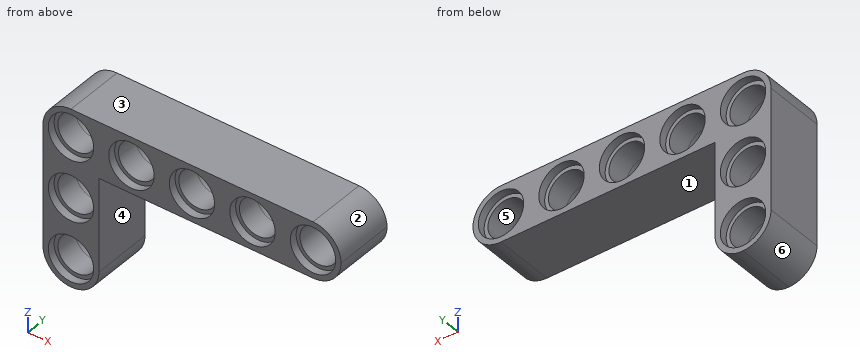
from build123d import *

# Parameters (mm, degrees)
F0_R     = 3
F1_DEPTH = 3.95
F0_R_2   = 2.499
F2_DEPTH = 2.95
F3_R     = 3.69999
F4_R     = 3
F4_W     = 7.4
F4_H     = 7.4
F5_DEPTH = 7.9
F7_R     = 3.69999
F8_R     = 3.7


# Not quite as in the source:
# - a fillet or chamfer is up to 0.001 mm smaller than in the source, because OpenCascade refuses the exact size


with BuildPart() as f1:
    # F0 (on Front) → F1 (new body, symmetric)
    with BuildSketch(Plane.XZ):
        Polygon((19.7, -3.7), (19.7, 3.7), (-19.7, 3.7), (-19.7, -3.7), (-19.7, -19.7), (-12.3, -19.7), (-12.3, -3.7), align=None)
        with Locations((-16, -16)):
            Circle(F0_R, mode=Mode.SUBTRACT)
        with Locations((-16, -8)):
            Circle(F0_R, mode=Mode.SUBTRACT)
        with Locations((-16, 0)):
            Circle(F0_R, mode=Mode.SUBTRACT)
        with Locations((-8, 0)):
            Circle(F0_R, mode=Mode.SUBTRACT)
        Circle(F0_R, mode=Mode.SUBTRACT)
        with Locations((8, 0)):
            Circle(F0_R, mode=Mode.SUBTRACT)
        with Locations((16, 0)):
            Circle(F0_R, mode=Mode.SUBTRACT)
    extrude(amount=F1_DEPTH, both=True)

    # F0 (on Front) → F2 (join, symmetric)
    with BuildSketch(Plane.XZ):
        with Locations((-16, -16)):
            Circle(F0_R)
        with Locations((-16, -16)):
            Circle(F0_R_2, mode=Mode.SUBTRACT)
        with Locations((-16, -8)):
            Circle(F0_R)
        with Locations((-16, -8)):
            Circle(F0_R_2, mode=Mode.SUBTRACT)
        with Locations((-16, 0)):
            Circle(F0_R)
        with Locations((-16, 0)):
            Circle(F0_R_2, mode=Mode.SUBTRACT)
        with Locations((-8, 0)):
            Circle(F0_R)
        with Locations((-8, 0)):
            Circle(F0_R_2, mode=Mode.SUBTRACT)
        Circle(F0_R)
        Circle(F0_R_2, mode=Mode.SUBTRACT)
        with Locations((8, 0)):
            Circle(F0_R)
        with Locations((8, 0)):
            Circle(F0_R_2, mode=Mode.SUBTRACT)
        with Locations((16, 0)):
            Circle(F0_R)
        with Locations((16, 0)):
            Circle(F0_R_2, mode=Mode.SUBTRACT)
    extrude(amount=F2_DEPTH, both=True)

    # F3 (radius 3.7 in the source; OpenCascade refuses exactly that, so slightly less here)
    f3_edges = [f1.edges().sort_by_distance(p)[0] for p in [
        (19.7, 0, 3.7),
        (19.7, 0, -3.7),
    ]]
    fillet(f3_edges, radius=F3_R)

    # F7 (radius 3.7 in the source; OpenCascade refuses exactly that, so slightly less here)
    f7_edges = [f1.edges().sort_by_distance(p)[0] for p in [
        (-12.3, 0, -19.7),
        (-19.7, 0, -19.7),
    ]]
    fillet(f7_edges, radius=F7_R)

    # F8
    f8_edges = [f1.edges().sort_by_distance(p)[0] for p in [
        (-19.7, 0, 3.7),
    ]]
    fillet(f8_edges, radius=F8_R)


with BuildPart() as f5:
    # F4 (on face) → F5 (new body)
    with BuildSketch(Plane.XZ.offset(3.95)):
        Polygon((-12.3, -19.7), (-12.3, -3.7), (-19.7, -3.7), (-19.7, -12.3), (-19.7, -19.7), align=None)
        with Locations((-16, -16)):
            Circle(F4_R, mode=Mode.SUBTRACT)
        with Locations((-16, -8)):
            Circle(F4_R, mode=Mode.SUBTRACT)
        with Locations((-23.4, -16)):
            Rectangle(F4_W, F4_H)
    extrude(amount=F5_DEPTH)


solid = f1.part
Verification items for the finished model (mm, model axes). Face numbers are marked on the shaded views. A direction names the side the tool comes from. Round coordinates to 2 decimals unless told otherwise and drop trailing zeros. Write each loop counter-clockwise with the first axis right and the second up, starting at its lowest first coordinate (ties: lowest second). Pieces come first, ordered by that corner, then holes.
(1) Depth check by flat-ended pin: pin 1 Ø6.5 at (x, z) = (0, 0) entering from +Y; pin 2 Ø5.5 at (x, z) = (16, 0) entering from -Y; pin 3 Ø1 at (y, z) = (0.5, -16.5) entering from +X. Enter the tip coordinate at first touch or a pass-through.
Returned:
pin 1: stops at y = 3.95
pin 2: stops at y = -2.95
pin 3: stops at x = -12.3
(2) Access from +Z, -Z, +X, -X, +Y, -Y to the whole of each face (thin tool, end or side, straight path). Record for the marked faces 1 and 2.
Returned:
face 1: -Z, +X, +Y, -Y
face 2: +Z, +X, +Y, -Y
(3) Section check A-A (y = -1). Give the number of separate pieces and of enclosed holes in the cut face, plus the area to 3 significant figures.
Returned:
separate pieces: 1
enclosed holes: 7
area: 258 mm2
(4) Section check B-B (x = -8). Enter the section's corners in (y, z), plus the area to 3 significant figures.
Returned:
outline: (-3.95, -3.7) - (3.95, -3.7) - (3.95, -3) - (2.95, -3) - (2.95, -2.5) - (-2.95, -2.5) - (-2.95, -3) - (-3.95, -3) - close; (-3.95, 3) - (-2.95, 3) - (-2.95, 2.5) - (2.95, 2.5) - (2.95, 3) - (3.95, 3) - (3.95, 3.7) - (-3.95, 3.7) - close
area: 17.0 mm2
(5) Section check C-C (z = -8). Enter the section's corners in (x, y), plus the area to 3 significant figures.
Returned:
outline: (-19.7, -3.95) - (-19, -3.95) - (-19, -2.95) - (-18.5, -2.95) - (-18.5, 2.95) - (-19, 2.95) - (-19, 3.95) - (-19.7, 3.95) - close; (-13.5, -2.95) - (-13, -2.95) - (-13, -3.95) - (-12.3, -3.95) - (-12.3, 3.95) - (-13, 3.95) - (-13, 2.95) - (-13.5, 2.95) - close
area: 17.0 mm2
(6) Material ranges on line 1 (Z direction, x = -16, y = -3.35); line 2 (Z direction, x = 0, y = 3.65); line 3 (X direction, y = 3.5, z = 1.75), recorded low to high.
Returned:
line 1: z = -19.7 to -19, -13 to -11, -5 to -3, 3 to 3.7
line 2: z = -3.7 to -3, 3 to 3.7
line 3: x = -19.26 to -18.44, -13.56 to -10.44, -5.56 to -2.44, 2.44 to 5.56, 10.44 to 13.56, 18.44 to 19.26
(7) Mould release check, pull along X, two halves, no side actions. Record for the marked faces 3, 4, 5 and 6: pulls with the +X half, pulls with the -X half, needs draft (parallel to the pull), parting line crosses it, or undercut.
Returned:
face 3: needs draft
face 4: pulls with the +X half
face 5: undercut
face 6: pulls with the -X half
